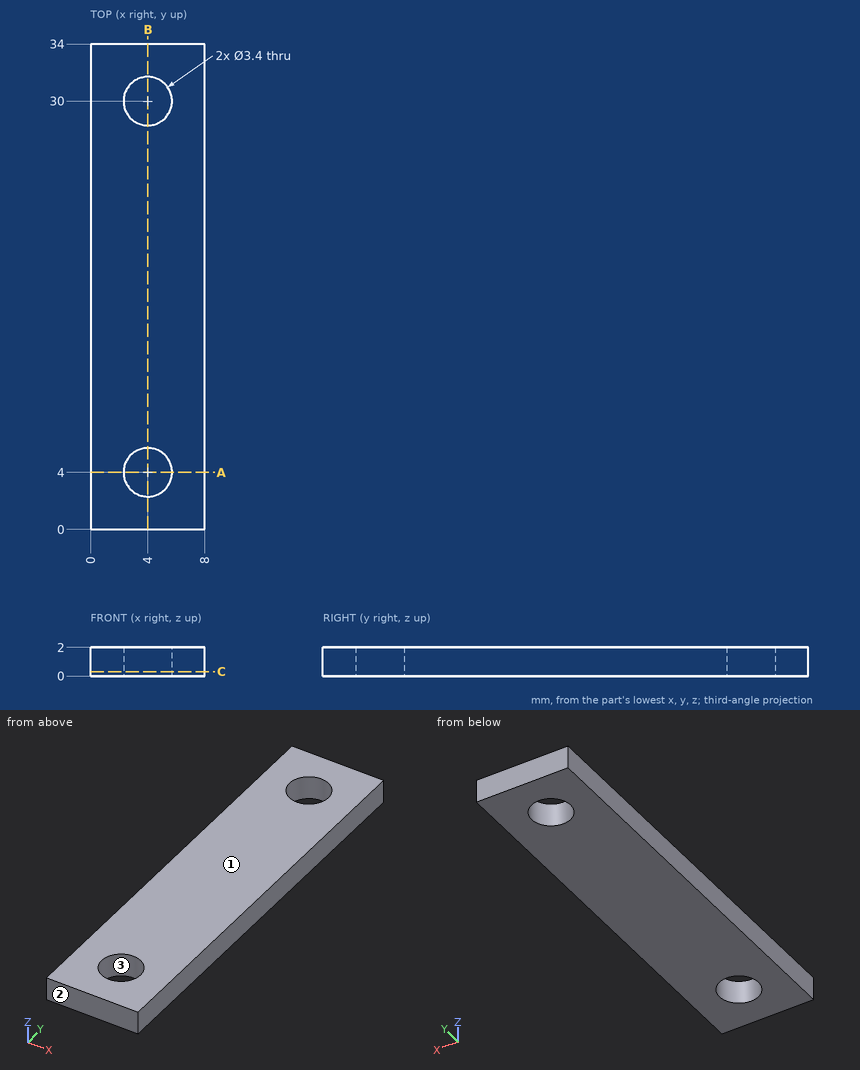
Study the drawing (mm; zero at the part's minimum x, y, z) and answer. Give positions to 0.01 mm unless a question says otherwise; leave off trailing zeros. Loops run counter-clockwise (first coordinate to the right, second up) from the corner with the lowest first, then second, coordinate; pieces in that order, holes last. Notation, with made-up numbers: (54, 16) -> (100, 16) arc R27 cw to (100, 44) -> close; hole circle Ø5 at (62, 33.25). An arc over 180 degrees is marked (long way). Use a Markdown table: item, result. Add a question column.
1) This flat-tipped pin is pushed along its axis until it touches: P1, Ø4.5, axis at x = 4, y = 4, coming from the +Z side. Where does it stop, or does it pass through?
2) The part is cut by section C-C, the plane z = 0.3. Determine the outline of the cut face in (x, y).
3) The part is cut by section A-A, the plane y = 4. Determine the outline of the cut face in (x, z), plus the area to 3 significant figures.
4) For a pull along Y with two mould halves and no side action, classify the marked faces 1, 2 and 3 as +Y half, -Y half, draft (parallel to the pull), parting line (faces both ways), or undercut.
5) Consider line 1 along Y through (x, z) = (4, 1.3); line 2 along Y through (x, z) = (3, 0.8); line 3 along X through (y, z) = (29, 1.8). Determine where each line is inside the solid, lowest interval first.
6) The part is cut by section B-B, the plane x = 4. Determine the outline of the cut face in (y, z), plus the area to 3 significant figures.
Reported:
| question | item | result |
|---|---|---|
| 1 | P1 | stops at z = 2 |
| 2 | outline | (0, 0) -> (8, 0) -> (8, 34) -> (0, 34) -> close; hole circle Ø3.4 at (4, 4); hole circle Ø3.4 at (4, 30) |
| 3 | outline | (0, 0) -> (2.3, 0) -> (2.3, 2) -> (0, 2) -> close; (5.7, 0) -> (8, 0) -> (8, 2) -> (5.7, 2) -> close |
| 3 | area | 9.20 mm^2 |
| 4 | face 1 | draft |
| 4 | face 2 | -Y half |
| 4 | face 3 | undercut |
| 5 | line 1 | y = 0 to 2.3, 5.7 to 28.3, 31.7 to 34 |
| 5 | line 2 | y = 0 to 2.63, 5.37 to 28.63, 31.37 to 34 |
| 5 | line 3 | x = 0 to 2.63, 5.37 to 8 |
| 6 | outline | (0, 0) -> (2.3, 0) -> (2.3, 2) -> (0, 2) -> close; (5.7, 0) -> (28.3, 0) -> (28.3, 2) -> (5.7, 2) -> close; (31.7, 0) -> (34, 0) -> (34, 2) -> (31.7, 2) -> close |
| 6 | area | 54.4 mm^2 |
